from build123d import *

# Parameters (mm, degrees)
SKETCH_1_W          = 15
SKETCH_1_H          = 8
SKETCH_1_R          = 0.85
EXTRUDE_1_DEPTH     = 2
SKETCH_2_R          = 1.95
EXTRUDE_2_DEPTH     = 20
SKETCH_3_R          = 1.25
CUT_EXTRUDE_1_DEPTH = 10


with BuildPart() as part:
    # 草图1 → 凸台-拉伸1 (new body)
    with BuildSketch(Plane(origin=(0, 0, 0), x_dir=(1, 0, 0), z_dir=(0, 1, 0))):
        with Locations((7.5, 4)):
            Rectangle(SKETCH_1_W, SKETCH_1_H)
        with Locations(Location((2.5, 4, 0), (0, 0, 270))):
            Circle(SKETCH_1_R, mode=Mode.SUBTRACT)
        with Locations(Location((12.5, 4, 0), (0, 0, 90))):
            Circle(SKETCH_1_R, mode=Mode.SUBTRACT)
    extrude(amount=EXTRUDE_1_DEPTH)

    # 草图2 → 凸台-拉伸2 (add)
    with BuildSketch(Plane(origin=(0, 2, 0), x_dir=(1, 0, 0), z_dir=(0, 1, 0))):
        with Locations(Location((7.5, 4, 0), (0, 0, 90))):
            Circle(SKETCH_2_R)
    extrude(amount=EXTRUDE_2_DEPTH)

    # 草图3 → 切除-拉伸1 (cut)
    with BuildSketch(Plane(origin=(0, 22, 0), x_dir=(1, 0, 0), z_dir=(0, 1, 0))):
        with Locations(Location((7.5, 4, 0), (0, 0, 270))):
            Circle(SKETCH_3_R)
    extrude(amount=-CUT_EXTRUDE_1_DEPTH, mode=Mode.SUBTRACT)


solid = part.part
Read the model definition and answer for the solid it produces. Units are mm, in the model's axes. A direction names the side the tool comes from. Coordinates: 2 decimals unless noted, no trailing zeros. Loops run counter-clockwise (first coordinate to the right, second up) from the corner with the lowest first, then second, coordinate; pieces in that order, holes last. Notation, with made-up numbers: (43, 21.25) -> (48, 21.25) arc R16 ccw to (48, 27.25) -> close; hole circle Ø5 at (44.5, -27). An arc over 180 degrees is marked (long way). Write item = value, one per line. Start each with the question number.
1) The part is cut by section A-A, the plane x = 2.5. Determine the outline of the cut face in (y, z).
2) Find the intervals of material crossed by L1, parallel to X at y = 0.5, z = -4; L2, parallel to X at y = 14.25, z = -4; L3, parallel to Z at x = 12.5, y = 0.7, in increasing order. Write a range as from..to.
3) The part is cut by section D-D, the plane y = 14. Determine the outline of the cut face in (x, z), plus the area to 3 significant figures.
4) Given P1, Ø2, axis at x = 2.5, z = -4, coming from the +Y side; P2, Ø0.8, axis at x = 7, z = -4.5, coming from the +Y side; P3, Ø2, axis at y = 10, z = -5, coming from the +X side, each flat-ended and moving along its own axis, determine where each tip first touches the part or whether it passes through.
5) The part is cut by section C-C, the plane x = 7.5. Determine the outline of the cut face in (y, z).
6) The part is cut by section B-B, the plane z = -4. Determine the outline of the cut face in (x, y).
7) The mould has two halves that part along X. Classify faces 3 (the face through (6.182, 11.86, -2.563)), 4 (the face through (11.657, 0.986, -3.889)), 5 (the face through (7, 0, -4)): pulls with the +X half, pulls with the -X half, needs draft (parallel to the pull), parting line crosses it, or undercut.
8) For faces 1 (the face through (6.28, 17.07, -4.27)), 2 (the face through (7, 1, -8)), determine the directions among +Z, -Z, +X, -X, +Y, -Y from which every point of the face is accessible in a straight line to the end or side of a thin tool.
Result:
q1.outline = (0, -8) -> (2, -8) -> (2, -4.85) -> (0, -4.85) -> close; (0, -3.15) -> (2, -3.15) -> (2, 0) -> (0, 0) -> close
q2.L1 = 0..1.65, 3.35..11.65, 13.35..15
q2.L2 = 5.55..6.25, 8.75..9.45
q2.L3 = -8..-4.85, -3.15..0
q3.outline = circle Ø3.9 at (7.5, -4); hole circle Ø2.5 at (7.5, -4)
q3.area = 7.04 mm²
q4.P1 = 2
q4.P2 = 12
q4.P3 = 9.45
q5.outline = (0, -8) -> (2, -8) -> (2, -5.95) -> (22, -5.95) -> (22, -5.25) -> (12, -5.25) -> (12, -2.75) -> (22, -2.75) -> (22, -2.05) -> (2, -2.05) -> (2, 0) -> (0, 0) -> close
q6.outline = (0, 0) -> (1.65, 0) -> (1.65, 2) -> (0, 2) -> close; (3.35, 0) -> (11.65, 0) -> (11.65, 2) -> (9.45, 2) -> (9.45, 22) -> (8.75, 22) -> (8.75, 12) -> (6.25, 12) -> (6.25, 22) -> (5.55, 22) -> (5.55, 2) -> (3.35, 2) -> close; (13.35, 0) -> (15, 0) -> (15, 2) -> (13.35, 2) -> close
q7.face_3 = parting line crosses it
q7.face_4 = undercut
q7.face_5 = needs draft
q8.face_1 = +Y
q8.face_2 = -Z, +X, -X, +Y, -Y
